Design review of the part shown in the three views and the two pictorial views. Dimensions are in mm from the part's minimum x, y and z. A direction names the side the tool comes from. Give positions to 0.01 mm unless a question says otherwise; leave off trailing zeros. Loops run counter-clockwise (first coordinate to the right, second up) from the corner with the lowest first, then second, coordinate; pieces in that order, holes last. Notation, with made-up numbers: (23.5, 68.5) -> (62.5, 68.5) arc R14 cw to (62.5, 82.5) -> close; hole circle Ø3 at (81, 16.25). An arc over 180 degrees is marked (long way). Use CSV: the item, a comma, the result in double quotes. Start each with the question number.
Item 1: Wall thickness on line 1 along Y through (x, z) = (15, 3.5); line 2 along Z through (x, y) = (106, 20.5); line 3 along Z through (x, y) = (89.5, 34) (1 decimal): over which ranges is each line inside the solid? List them lowest first. Write a range as from..to.
Item 2: We need section D-D (z = 13). State the section outline as (x, y) points.
Item 3: Clearance check with flat-ended pins moving along their axes: pin 1 (18 mm diameter, centred on x = 66, z = 38, fed in from +Y); pin 2 (12 mm diameter, centred on y = 61.5, z = 73.5, fed in from -X); pin 3 (24 mm diameter, centred on x = 58.5, y = 42.5, fed in from +Z) (1 decimal). State where each tip first meets the part, or that it passes through.
Item 4: For the marked faces 5, 6, 7 and 8, list the 3-axis set-ups (+Z, -Z, +X, -X, +Y, -Y) from which the entire face can be reached by the end or side of a thin tool; tool diameter is ignored.
Item 5: The part is to be moulded in two halves that separate along X. For the marked faces 1, 2, 3 and 4, say which applies: +X half, -X half, draft (parallel to the pull), parting line (faces both ways), or undercut.
Item 6: We need section C-C (x = 90). State the section outline as (y, z) points, plus the area to 3 significant figures.
Item 7: We need section A-A (y = 15). State the section outline as (x, z) points.
Item 8: We need section B-B (y = 68). State the section outline as (x, z) points.
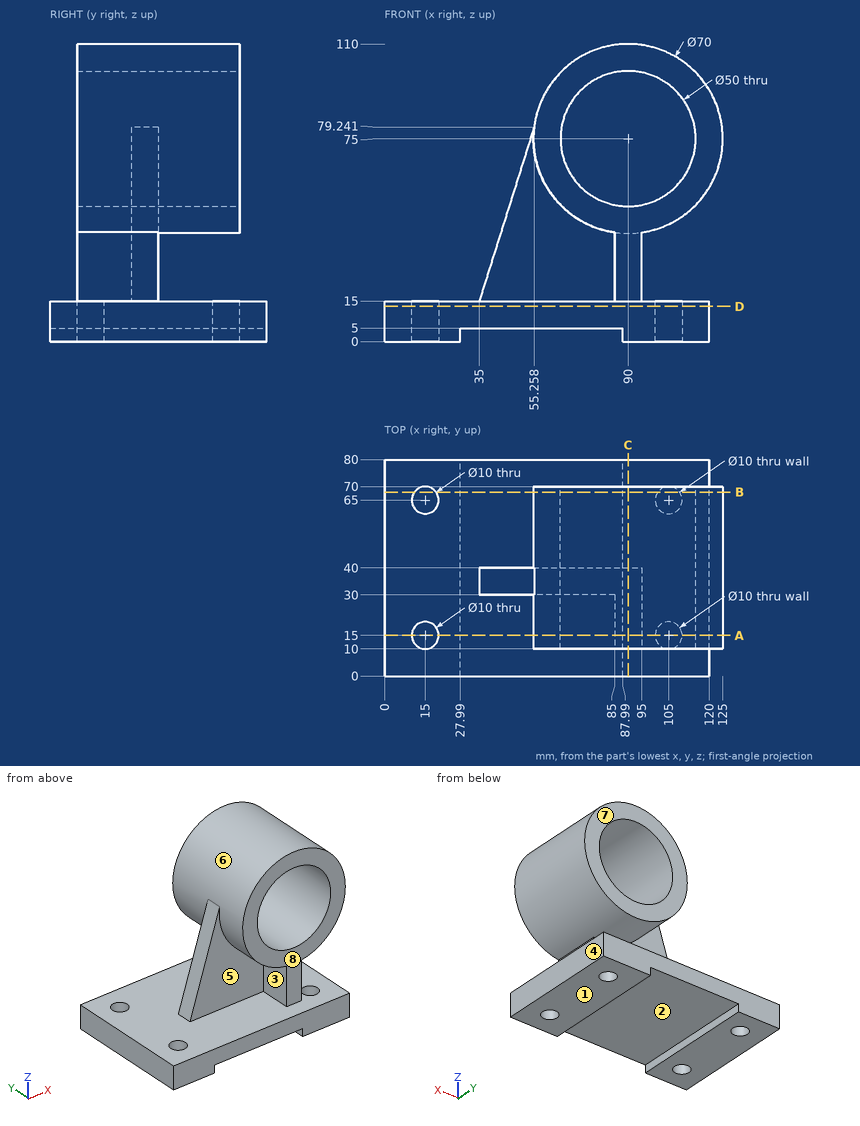
Results found:
1,line 1,"0..10, 20..60, 70..80"
1,line 2,"0..15, 43.87..55.79, 94.21..106.13"
1,line 3,"0..50, 100..110"
2,outline,"(0, 0) -> (120, 0) -> (120, 80) -> (0, 80) -> close; hole circle Ø10 at (15, 15); hole circle Ø10 at (15, 65); hole circle Ø10 at (105, 15); hole circle Ø10 at (105, 65)"
3,pin 1,"y = 40"
3,pin 2,"x = 55"
3,pin 3,"z = 104.1"
4,face 5,"-X, -Y"
4,face 6,"none"
4,face 7,"+Z, +X, -X, +Y"
4,face 8,"+Z, +X, -X, -Y"
5,face 1,"draft"
5,face 2,"undercut"
5,face 3,"-X half"
5,face 4,"+X half"
6,outline,"(0, 0) -> (80, 0) -> (80, 15) -> (40, 15) -> (40, 40) -> (70, 40) -> (70, 50) -> (10, 50) -> (10, 15) -> (0, 15) -> close; (10, 100) -> (70, 100) -> (70, 110) -> (10, 110) -> close"
6,area,"3,150 mm²"
7,outline,"(0, 0) -> (10, 0) -> (10, 15) -> (0, 15) -> close; (20, 0) -> (27.99, 0) -> (27.99, 5) -> (87.99, 5) -> (87.99, 0) -> (100, 0) -> (100, 15) -> (95, 15) -> (95, 40.36) arc R35 ccw (long way) to (85, 40.36) -> (85, 15) -> (20, 15) -> close; (110, 0) -> (120, 0) -> (120, 15) -> (110, 15) -> close; hole circle Ø50 at (90, 75)"
8,outline,"(0, 0) -> (11, 0) -> (11, 15) -> (0, 15) -> close; (19, 0) -> (27.99, 0) -> (27.99, 5) -> (87.99, 5) -> (87.99, 0) -> (101, 0) -> (101, 15) -> (19, 15) -> close; circle Ø70 at (90, 75); (109, 0) -> (120, 0) -> (120, 15) -> (109, 15) -> close; hole circle Ø50 at (90, 75)"
